Input: part model. Units: mm. Frame: model coordinates. A direction names the side the tool comes from. Coordinates: 2 decimals unless noted, no trailing zeros. Order: outer loops, then holes, each group sorted by start corner. A loop starts at its lowest first (then second) coordinate and runs counter-clockwise, first axis right, second up. Notation, with made-up numbers: (-6, 49.5) - (0, 49.5) arc R10 cw to (0, 67.5) - close; hole circle Ø10 at (14, 55.25). An arc over 180 degrees is marked (long way). Use a Markdown table: item, result. Add a question column.
from build123d import *

# Parameters (mm, degrees)
F1_DEPTH       = 37
F2_DEPTH       = 35.5
F4_D           = 4
F4_DEPTH       = 5
F4_CBORE_D     = 5
F4_CBORE_DEPTH = 1
F4_TIP         = 1.2017212381


with BuildPart() as f1:
    # F0 (on Front) → F1 (new body, symmetric)
    with BuildSketch(Plane.XZ):
        Polygon((-1.0269926464, -1.716183587), (0, 0), (-11.4757237546, 6.8672629181), (-13.0274063785, 5.4650624927), (-11.7402686883, 4.6948180079), (-2.3141303366, -0.9459391022), align=None)
    extrude(amount=F1_DEPTH, both=True)

    # F0 (on Front) → F2 (join, symmetric)
    with BuildSketch(Plane.XZ):
        Polygon((-2.3141303366, -3.2766920766), (-2.3141303366, -0.9459391022), (-11.7402686883, 4.6948180079), (-11.7402686883, 2.3640650335), align=None)
    extrude(amount=F2_DEPTH, both=True)

    # F4
    with Locations(Plane(origin=(0, 0, 0), x_dir=(0.8580917935, 0, -0.5134963232), z_dir=(0.5134963232, 0, 0.8580917935))):
        with Locations((-6.6867693185, 20), (-6.6867693185, 0), (-6.6867693185, -20)):
            CounterBoreHole(F4_D / 2, F4_CBORE_D / 2, F4_CBORE_DEPTH, depth=F4_DEPTH)
            with Locations((0, 0, -(F4_DEPTH + F4_TIP / 2))):  # 118° drill point
                Cone(0, F4_D / 2, F4_TIP, mode=Mode.SUBTRACT)


solid = f1.part
1) Material intervals for L1, parallel to Y at x = -7, z = 1; L2, parallel to Y at x = -6.25, z = 1.5; L3, parallel to Y at x = -11.5, z = 3.75, sorted ascending.
2) Cut plane A-A (y = -25.5). Return the cut outline in (x, z).
3) Reachability of faces 4 (the flat face through (-7, 35.5, 1)), 5 (the flat face through (-7, -35.5, 1)), 6 (the flat face through (-5, -0.5, -1.67)) from +Z, -Z, +X, -X, +Y, -Y: full face, straight path, thin tool, end or side. Return the list, or none.
4) Cut plane B-B (x = -10.5). Return the cut outline in (y, z).
5) Contact query for flat-ended pins moving along their axis: P1, Ø2.5, axis at x = -6.5, z = 0, coming from the -Y side; P2, Ø1.9, axis at y = -8.5, z = -1.5, coming from the +X side; P3, Ø1.9, axis at y = -2.5, z = 4, coming from the -X side. Output: stop coordinate, or through.
6) Pull-direction query (X, two-part tool) for faces 1 (the cylindrical face through (-7.693, -1.521, 4.029)), 2 (the flat face through (-11.74, 0, 4)), 3 (the flat face through (-0.52, -0.52, -0.87)); classes: pulls with the +X half, pulls with the -X half, needs draft (parallel to the pull), parting line crosses it, or undercut.
Computed:
| question | item | result |
|---|---|---|
| 1 | L1 | y = -35.5 to -21.99, -18.01 to -1.99, 1.99 to 18.01, 21.99 to 35.5 |
| 1 | L2 | y = -37 to -21.92, -18.08 to -1.92, 1.92 to 18.08, 21.92 to 37 |
| 1 | L3 | y = -35.5 to 35.5 |
| 2 | outline | (-13.03, 5.47) - (-11.74, 4.69) - (-11.74, 2.36) - (-2.31, -3.28) - (-2.31, -0.95) - (-1.03, -1.72) - (0, 0) - (-11.48, 6.87) - close |
| 3 | face 4 | -Z, -X, +Y |
| 3 | face 5 | -Z, -X, -Y |
| 3 | face 6 | -Z, -X, +Y, -Y |
| 4 | outline | (-37, 3.95) - (-35.5, 3.95) - (-35.5, 1.62) - (35.5, 1.62) - (35.5, 3.95) - (37, 3.95) - (37, 6.28) - (-37, 6.28) - close |
| 5 | P1 | stops at y = -35.5 |
| 5 | P2 | stops at x = -0.33 |
| 5 | P3 | stops at x = -12.17 |
| 6 | face 1 | undercut |
| 6 | face 2 | pulls with the -X half |
| 6 | face 3 | pulls with the +X half |
